Geometry: final body of the model. Coordinates: model frame, mm. A direction names the side the tool comes from. Give positions to 0.01 mm unless a question says otherwise; leave off trailing zeros. Write each loop counter-clockwise with the first axis right and the second up, starting at its lowest first coordinate (ties: lowest second). Pieces come first, ordered by that corner, then holes. Notation, with made-up numbers: (-40, 5.5) - (-16, 5.5) arc R18 cw to (-16, 9.5) - close; hole circle Ø7 at (2.5, -39.75). An arc over 180 degrees is marked (long way). Return JSON: item names as keys, results as strings.
from build123d import *

# Parameters (mm, degrees)
F0_R     = 66.75
F1_DEPTH = 12
F2_R     = 56.75
F2_R_2   = 51.75
F3_DEPTH = 35
F6_DEPTH = 12
F7_R     = 5.5
F8_DEPTH = 12


with BuildPart() as f1:
    # F0 (on Top) → F1 (new body)
    with BuildSketch(Plane.XY):
        Circle(F0_R)
    extrude(amount=F1_DEPTH)

    # F2 (on face) → F3 (join)
    with BuildSketch(Plane.XY.offset(12)):
        Circle(F2_R)
        Circle(F2_R_2, mode=Mode.SUBTRACT)
    extrude(amount=F3_DEPTH)

    # F5 (on Top) → F6 (cut)
    with BuildSketch(Plane.XY):
        with BuildLine():
            ThreePointArc((-1.8982756668, 61.7208153664), (0, 59.8515), (1.8982756668, 61.7208153664))
            ThreePointArc((1.8982756668, 61.7208153664), (0, 61.75), (-1.8982756668, 61.7208153664))
        make_face()
        with BuildLine():
            ThreePointArc((-1.8982756668, 61.7208153664), (0, 61.75), (1.8982756668, 61.7208153664))
            ThreePointArc((1.8982756668, 61.7208153664), (1.8984439159, 61.7354072521), (1.8985, 61.75))
            ThreePointArc((1.8985, 61.75), (-0.0145927479, 63.6484439159), (-1.8982756668, 61.7208153664))
        make_face()
        with BuildLine():
            ThreePointArc((61.7208153664, 1.8982756668), (61.7427034105, 0.94925), (61.75, 0))
            ThreePointArc((61.75, 0), (61.7427034105, -0.94925), (61.7208153664, -1.8982756668))
            ThreePointArc((61.7208153664, -1.8982756668), (63.0820839356, -1.3527211976), (63.6485, 0))
            ThreePointArc((63.6485, 0), (63.0820839356, 1.3527211976), (61.7208153664, 1.8982756668))
        make_face()
        with BuildLine():
            ThreePointArc((61.7208153664, -1.8982756668), (61.7427034105, -0.94925), (61.75, 0))
            ThreePointArc((61.75, 0), (61.7427034105, 0.94925), (61.7208153664, 1.8982756668))
            ThreePointArc((61.7208153664, 1.8982756668), (59.8515, 0), (61.7208153664, -1.8982756668))
        make_face()
        with BuildLine():
            ThreePointArc((1.8985, -61.75), (1.8984439159, -61.7354072521), (1.8982756668, -61.7208153664))
            ThreePointArc((1.8982756668, -61.7208153664), (0, -61.75), (-1.8982756668, -61.7208153664))
            ThreePointArc((-1.8982756668, -61.7208153664), (-0.0145927479, -63.6484439159), (1.8985, -61.75))
        make_face()
        with BuildLine():
            ThreePointArc((-1.8982756668, -61.7208153664), (0, -61.75), (1.8982756668, -61.7208153664))
            ThreePointArc((1.8982756668, -61.7208153664), (0, -59.8515), (-1.8982756668, -61.7208153664))
        make_face()
        with BuildLine():
            ThreePointArc((-59.8515, 0), (-60.3972788024, 1.3320839356), (-61.7208153664, 1.8982756668))
            ThreePointArc((-61.7208153664, 1.8982756668), (-61.75, 0), (-61.7208153664, -1.8982756668))
            ThreePointArc((-61.7208153664, -1.8982756668), (-60.3972788024, -1.3320839356), (-59.8515, 0))
        make_face()
        with BuildLine():
            ThreePointArc((-61.7208153664, -1.8982756668), (-61.75, 0), (-61.7208153664, 1.8982756668))
            ThreePointArc((-61.7208153664, 1.8982756668), (-63.6485, 0), (-61.7208153664, -1.8982756668))
        make_face()
    extrude(amount=F6_DEPTH, mode=Mode.SUBTRACT)

    # F7 (on Top) → F8 (cut)
    with BuildSketch(Plane.XY):
        Circle(F7_R)
    extrude(amount=F8_DEPTH, mode=Mode.SUBTRACT)


solid = f1.part
Q1. Section query A-A, the plane x = 0. Return the cut outline in (y, z), plus the area to 3 significant figures.
Answer key:
{"outline": "(-66.75, 0) - (-63.65, 0) - (-63.65, 12) - (-66.75, 12) - close; (-59.85, 0) - (-5.5, 0) - (-5.5, 12) - (-51.75, 12) - (-51.75, 47) - (-56.75, 47) - (-56.75, 12) - (-59.85, 12) - close; (5.5, 0) - (59.85, 0) - (59.85, 12) - (56.75, 12) - (56.75, 47) - (51.75, 47) - (51.75, 12) - (5.5, 12) - close; (63.65, 0) - (66.75, 0) - (66.75, 12) - (63.65, 12) - close", "area": "1,730 mm^2"}
Q2. Section query C-C, the plane z = 20. Return the cut outline in (x, y).
Answer key:
{"outline": "circle Ø113.5 at (0, 0); hole circle Ø103.5 at (0, 0)"}
Q3. Material intervals for probe 1 along Z at (x, y) = (18, 5); probe 2 along Y at (x, z) = (26, 21.5); probe 3 along X at (y, z) = (7.5, 21.5), sorted ascending. Write a range as [from, to].
Answer key:
{"probe 1": "z = [0, 12]", "probe 2": "y = [-50.44, -44.74], [44.74, 50.44]", "probe 3": "x = [-56.25, -51.2], [51.2, 56.25]"}
Q4. Mould query, pull axis Y, two halves, no side actions, for faces 1 (the cylindrical face through (-52.97, -40.62, 5.92)), 2 (the flat face through (-1, -11, 12)), 3 (the flat face through (25, -46, 47)). Classes: pulls with the +Y half, pulls with the -Y half, needs draft (parallel to the pull), parting line crosses it, or undercut.
Answer key:
{"face 1": "parting line crosses it", "face 2": "undercut", "face 3": "needs draft"}
Q5. Set-up query: faces 4 (the cylindrical face through (-41.83, 38.35, 29.26)), 5 (the cylindrical face through (-1.19, -5.37, 5.92)). Return all of +Z, -Z, +X, -X, +Y, -Y with unobstructed straight access to the full face (end or side cutting, diameter ignored); none if empty.
Answer key:
{"face 4": "+Z", "face 5": "+Z, -Z"}
Q6. Section query B-B, the plane y = -20. Return the cut outline in (x, z), plus the area to 3 significant figures.
Answer key:
{"outline": "(-63.68, 0) - (63.68, 0) - (63.68, 12) - (53.11, 12) - (53.11, 47) - (47.73, 47) - (47.73, 12) - (-47.73, 12) - (-47.73, 47) - (-53.11, 47) - (-53.11, 12) - (-63.68, 12) - close", "area": "1,900 mm^2"}
Q7. Pin query (flat end, axial travel): P1, Ø1.5, axis at x = 45.5, z = 24.5, coming from the -Y side; P2, Ø2, axis at x = 48, z = 37, coming from the -Y side; P3, Ø1, axis at x = -42.5, z = 30, coming from the +Y side. Return the tip coordinate at first contact, or that it passes through.
Answer key:
{"P1": "stops at y = -34.9", "P2": "stops at y = -31.81", "P3": "stops at y = 38.16"}
Q8. Section query D-D, the plane x = -41. Return the cut outline in (y, z), plus the area to 3 significant figures.
Answer key:
{"outline": "(-52.67, 0) - (52.67, 0) - (52.67, 12) - (39.24, 12) - (39.24, 47) - (31.58, 47) - (31.58, 12) - (-31.58, 12) - (-31.58, 47) - (-39.24, 47) - (-39.24, 12) - (-52.67, 12) - close", "area": "1,800 mm^2"}
